from build123d import *

# Parameters (mm, degrees)
BOSS_EXTRUDE1_DEPTH     = 50
BOSS_EXTRUDE3_DEPTH     = 8
BOSS_EXTRUDE4_START     = 42
BOSS_EXTRUDE4_DEPTH     = 8
BOSS_EXTRUDE5_START     = -1
SKETCH1_6_R             = 25
SKETCH1_6_R_2           = 12.5
BOSS_EXTRUDE5_DEPTH     = 9
BOSS_EXTRUDE7_START     = 42
SKETCH1_8_R             = 25
BOSS_EXTRUDE7_DEPTH     = 9
CUT_EXTRUDE1_DEPTH      = 193.132564476
CUT_EXTRUDE1_DEPTH_BACK = 193.132564476
SKETCH1_10_R            = 12.5
CUT_EXTRUDE2_DEPTH      = 190.755469869
CUT_EXTRUDE2_DEPTH_BACK = 190.755469869
SKETCH2_R               = 7.5


with BuildPart() as part:
    # Sketch1 → Boss-Extrude1 (new body)
    with BuildSketch(Plane.XY):
        Polygon((26.59102299, 8), (149.554580342, 8), (175, 8), (175, 0), (0, 0), (0, 8), align=None)
    extrude(amount=BOSS_EXTRUDE1_DEPTH)

    # Sketch1<4> → Boss-Extrude3 (add)
    with BuildSketch(Plane.XY):
        with BuildLine():
            ThreePointArc((34.21809324, 11.532558512), (30.793735514, 8.926014798), (26.59102299, 8))
            Line((26.59102299, 8), (149.554580342, 8))
            ThreePointArc((149.554580342, 8), (145.422937943, 8.893434726), (142.029566102, 11.414093784))
            Line((142.029566102, 11.414093784), (106.332559555, 52.201264717))
            ThreePointArc((106.332559555, 52.201264717), (110.922089996, 44.531003426), (112.520023955, 35.736499176))
            ThreePointArc((112.520023955, 35.736499176), (78.908749097, 12.266391692), (68.45234833, 51.905102896))
            Line((68.45234833, 51.905102896), (34.21809324, 11.532558512))
        make_face()
    extrude(amount=BOSS_EXTRUDE3_DEPTH)

    # Sketch1<5> → Boss-Extrude4 (add)
    with BuildSketch(Plane.XY.offset(BOSS_EXTRUDE4_START)):
        with BuildLine():
            ThreePointArc((34.21809324, 11.532558512), (30.793735514, 8.926014798), (26.59102299, 8))
            Line((26.59102299, 8), (149.554580342, 8))
            ThreePointArc((149.554580342, 8), (145.422937943, 8.893434726), (142.029566102, 11.414093784))
            Line((142.029566102, 11.414093784), (106.332559555, 52.201264717))
            ThreePointArc((106.332559555, 52.201264717), (110.922089996, 44.531003426), (112.520023955, 35.736499176))
            ThreePointArc((112.520023955, 35.736499176), (78.908749097, 12.266391692), (68.45234833, 51.905102896))
            Line((68.45234833, 51.905102896), (34.21809324, 11.532558512))
        make_face()
    extrude(amount=BOSS_EXTRUDE4_DEPTH)

    # Sketch1<6> → Boss-Extrude5 (add)
    with BuildSketch(Plane.XY.offset(BOSS_EXTRUDE5_START)):
        with Locations((87.520023955, 35.736499176)):
            Circle(SKETCH1_6_R)
        with Locations((87.520023955, 35.736499176)):
            Circle(SKETCH1_6_R_2, mode=Mode.SUBTRACT)
    extrude(amount=BOSS_EXTRUDE5_DEPTH)

    # Sketch1<8> → Boss-Extrude7 (add)
    with BuildSketch(Plane.XY.offset(BOSS_EXTRUDE7_START)):
        with Locations((87.520023955, 35.736499176)):
            Circle(SKETCH1_8_R)
    extrude(amount=BOSS_EXTRUDE7_DEPTH)

    # Sketch1<10> → Cut-Extrude1 (cut, two sides: drawn at the far end of the back side and taken through both)
    with BuildSketch(Plane.XY.offset(-CUT_EXTRUDE1_DEPTH_BACK)):
        with Locations((87.520023955, 35.736499176)):
            Circle(SKETCH1_10_R)
    extrude(amount=CUT_EXTRUDE1_DEPTH + CUT_EXTRUDE1_DEPTH_BACK, mode=Mode.SUBTRACT)

    # Sketch2 → Cut-Extrude2 (cut, two sides: drawn at the far end of the back side and taken through both)
    with BuildSketch(Plane(origin=(0, 8, 0), x_dir=(1, 0, 0), z_dir=(0, 1, 0)).offset(-CUT_EXTRUDE2_DEPTH_BACK)):
        with Locations(Location((16, -25, 0), (0, 0, 270))):
            Circle(SKETCH2_R)
        with Locations(Location((159, -25, 0), (0, 0, 270))):
            Circle(SKETCH2_R)
    extrude(amount=CUT_EXTRUDE2_DEPTH + CUT_EXTRUDE2_DEPTH_BACK, mode=Mode.SUBTRACT)


solid = part.part
Model file for the job. Use its own axes, mm. A direction names the side the tool comes from. Give positions to 0.01 mm unless a question says otherwise; leave off trailing zeros. Order: outer loops, then holes, each group sorted by start corner. A loop starts at its lowest first (then second) coordinate and runs counter-clockwise, first axis right, second up. Notation, with made-up numbers: M 24,-24.5 L 82,-24.5 A25 ccw 82,11.5 Z; hole C -37,65.5 d4. An arc over 180 degrees is marked long. Put each result on its own line as item: value. Start each with the question number.
(1) Tool access for faces 1 (the face through (145.477, 8.869, 3.944)), 2 (the face through (84.266, 60.524, 47.437)), 3 (the face through (84.266, 60.524, 2.437)), 4 (the face through (30.849, 8.952, 3.944)), 5 (the face through (87, 23, 8)): list every direction of +Z, -Z, +X, -X, +Y, -Y with a clear straight run to the whole face (end or side of a thin tool).
(2) Band-saw the part on C-C on y = 46. Give the cut face in (x, z).
(3) Band-saw the part on A-A on x = 159. Give the cut face in (y, z), then the cut area to 3 significant figures.
(4) Pull direction Z, two halves, no side cores. Call faces 6 (the face through (93.29, 24.65, 46.44)), 7 (the face through (81, 11, 0)), 8 (the face through (81, 11, 50)), 9 (the face through (21.1, 3.9, 19.5)): released by +Z, released by -Z, zero draft, split by the parting line, or undercut.
(5) Band-saw the part on B-B on z = 25. Give the cut face in (x, y).
(6) Pin check, flat tips, straight feed: pin 1 Ø3 at (x, z) = (68.5, 4.5) entering from +Y; pin 2 Ø1 at (x, z) = (134, 38) entering from -Y; pin 3 Ø6 at (y, z) = (17, 8.5) entering from +X; pin 4 Ø5 at (x, z) = (64, 8.5) entering from +Y. Stop position of each tip, or through.
(7) Drill centre lines: L1, parallel to X at y = 5.25, z = 25; L2, parallel to X at y = 7.5, z = 21; L3, parallel to Z at x = 111.5, y = 18. Where is each one in solid material? Low to high. Write a range as [from, to].
Results below:
1. face 1: +Z, -Z, +X, +Y
1. face 2: +Z
1. face 3: -Z
1. face 4: +Z, -Z, -X, +Y
1. face 5: +X, -X, +Y
2. outline: M 63.45,0 L 64.72,0 L 64.72,-1 L 80.38,-1 L 80.38,8 L 63.45,8 Z; M 63.45,42 L 80.38,42 L 80.38,51 L 64.72,51 L 64.72,50 L 63.45,50 Z; M 94.66,-1 L 110.32,-1 L 110.32,0 L 111.76,0 L 111.76,8 L 94.66,8 Z; M 94.66,42 L 111.76,42 L 111.76,50 L 110.32,50 L 110.32,51 L 94.66,51 Z
3. outline: M 0,0 L 8,0 L 8,17.5 L 0,17.5 Z; M 0,32.5 L 8,32.5 L 8,50 L 0,50 Z
3. area: 280 mm2
4. face 6: zero draft
4. face 7: released by -Z
4. face 8: released by +Z
4. face 9: undercut
5. outline: M 0,0 L 8.5,0 L 8.5,8 L 0,8 Z; M 23.5,0 L 151.5,0 L 151.5,8 L 23.5,8 Z; M 166.5,0 L 175,0 L 175,8 L 166.5,8 Z
6. pin 1: stops at y = 53.57
6. pin 2: stops at y = 0
6. pin 3: stops at x = 139.73
6. pin 4: stops at y = 49.54
7. L1: x = [0, 8.5], [23.5, 151.5], [166.5, 175]
7. L2: x = [0, 9.66], [22.34, 152.66], [165.34, 175]
7. L3: z = [0, 8], [42, 50]
